Part model, mm, in its own coordinate system. Face numbers are marked on the shaded views. A direction names the side the tool comes from. Round coordinates to 2 decimals unless told otherwise and drop trailing zeros. Write each loop counter-clockwise with the first axis right and the second up, starting at its lowest first coordinate (ties: lowest second). Pieces come first, ordered by that corner, then holes. Notation, with made-up numbers: (40, 5) -> (97, 5) arc R19 cw to (97, 12) -> close; hole circle Ø10 at (65.5, -20.75). An arc over 180 degrees is marked (long way). Use CSV: the item, a comma, the result in double quotes. Start each with the question number.
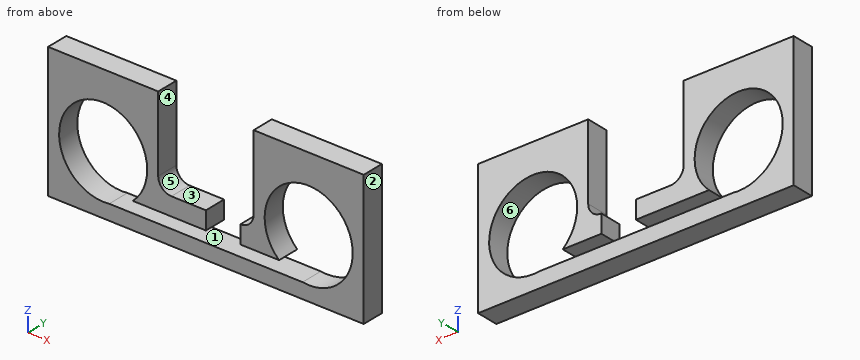
```python
from build123d import *

# Parameters (mm, degrees)
F0_W     = 273.05
F0_H     = 114.3
F1_DEPTH = 19.05
F2_R     = 38.1
F3_DEPTH = 25.4
F5_DEPTH = 25.4
F7_DEPTH = 25.4


with BuildPart() as f1:
    # F0 (on Front) → F1 (new body)
    with BuildSketch(Plane.XZ):
        with Locations((136.525, 57.15)):
            Rectangle(F0_W, F0_H)
    extrude(amount=F1_DEPTH)

    # F2 (on face) → F3 (cut)
    with BuildSketch(Plane.XZ.offset(19.05)):
        with Locations((225.425, 50.8)):
            Circle(F2_R)
        with Locations((47.625, 50.8)):
            Circle(F2_R)
    extrude(amount=-F3_DEPTH, mode=Mode.SUBTRACT)

    # F4 (on face) → F5 (cut)
    with BuildSketch(Plane.XZ.offset(19.05)):
        with BuildLine():
            Line((177.8, 114.3), (95.25, 114.3))
            Line((95.25, 114.3), (95.25, 49.53))
            ThreePointArc((95.25, 49.53), (98.597769, 41.447769), (106.68, 38.1))
            Line((106.68, 38.1), (166.37, 38.1))
            ThreePointArc((166.37, 38.1), (174.452231, 41.447769), (177.8, 49.53))
            Line((177.8, 49.53), (177.8, 114.3))
        make_face()
    extrude(amount=-F5_DEPTH, mode=Mode.SUBTRACT)

    # F6 (on face) → F7 (cut)
    with BuildSketch(Plane.XZ.offset(19.05)):
        Polygon((166.37, 22.5902), (166.37, 38.1), (136.525, 38.1), (136.525, 22.5902), (54.541018, 22.5902), (42.362412, 13.0652), (230.687588, 13.0652), (218.817472, 22.5902), align=None)
    extrude(amount=-F7_DEPTH, mode=Mode.SUBTRACT)


solid = f1.part
```
1. Band-saw the part on D-D (x = 182). List the corners of the cut face in (y, z).
2. Band-saw the part on C-C (y = -6.25). List the corners of the cut face in (x, z) (3 decimals), then the cut area to 3 significant figures.
3. Pull direction Z, two halves, no side cores. Call the marked faces 4, 5 and 6: released by +Z, released by -Z, zero draft, split by the parting line, or undercut.
4. Drill centre lines: line 1 along X through (y, z) = (-9.5, 50.8) (3 decimals); line 2 along X through (y, z) = (-4.5, 37) (3 decimals); line 3 along Z through (x, y) = (126.5, -4). Where is each one in solid material? Low to high. Write a range as [from, to].
5. Band-saw the part on B-B (z = 52). List the corners of the cut face in (x, y), then the cut area to 3 significant figures.
6. Flat gauge pins, fed straight in: pin 1 (4 mm diameter, centred on y = -17, z = 18, fed in from -X); pin 2 (9.5 mm diameter, centred on x = 154, y = -5.5, fed in from +Z); pin 3 (5.5 mm diameter, centred on x = 118.5, y = -5, fed in from +Z); pin 4 (8 mm diameter, centred on x = 166, y = -13, fed in from +Z). Where does each tip first touch, or does it go through?
7. Which spindle directions (+Z, -Z, +X, -X, +Y, -Y) get a long thin tool onto all of the face, cutting with end or side? Do the marked faces 1, 2 and 3. Say none if no direction does.
8. Band-saw the part on A-A (x = 116). List the corners of the cut face in (y, z).
Answers below:
1,outline,"(-19.05, 0) -> (0, 0) -> (0, 13.07) -> (-19.05, 13.07) -> close; (-19.05, 22.59) -> (0, 22.59) -> (0, 114.3) -> (-19.05, 114.3) -> close"
2,outline,"(0, 0) -> (273.05, 0) -> (273.05, 114.3) -> (177.8, 114.3) -> (177.8, 49.53) arc R11.43 cw to (166.37, 38.1) -> (166.37, 22.59) -> (199.816, 22.59) arc R38.1 cw (long way) to (220.162, 13.065) -> (52.888, 13.065) arc R38.1 cw (long way) to (73.234, 22.59) -> (136.525, 22.59) -> (136.525, 38.1) -> (106.68, 38.1) arc R11.43 cw to (95.25, 49.53) -> (95.25, 114.3) -> (0, 114.3) -> close"
2,area,"14,000 mm^2"
3,face 4,"zero draft"
3,face 5,"released by +Z"
3,face 6,"undercut"
4,line 1,"x = [0, 9.525], [85.725, 95.25], [177.8, 187.325], [263.525, 273.05]"
4,line 2,"x = [0, 12.112], [83.138, 136.525], [166.37, 189.912], [260.938, 273.05]"
4,line 3,"z = [0, 13.07], [22.59, 38.1]"
5,outline,"(0, -19.05) -> (9.54, -19.05) -> (9.54, 0) -> (0, 0) -> close; (85.71, -19.05) -> (95.25, -19.05) -> (95.25, 0) -> (85.71, 0) -> close; (177.8, -19.05) -> (187.34, -19.05) -> (187.34, 0) -> (177.8, 0) -> close; (263.51, -19.05) -> (273.05, -19.05) -> (273.05, 0) -> (263.51, 0) -> close"
5,area,"727 mm^2"
6,pin 1,"stops at x = 0"
6,pin 2,"stops at z = 13.07"
6,pin 3,"stops at z = 38.1"
6,pin 4,"stops at z = 38.69"
7,face 1,"+Y, -Y"
7,face 2,"+Z, -Z, +X, +Y, -Y"
7,face 3,"+Z, +Y, -Y"
8,outline,"(-19.05, 0) -> (0, 0) -> (0, 13.07) -> (-19.05, 13.07) -> close; (-19.05, 22.59) -> (0, 22.59) -> (0, 38.1) -> (-19.05, 38.1) -> close"
